Autodesk Fusion 360 part; units mm, degrees
sketch "Sketch1" plane through (0, 0, 0) normal (0, 1, 0) x (1, 0, 0)
  line L0 (39.5, -25.25) -> (-39.5, -25.25)
  line L1 (-43, -21.75) -> (-43, 21.75)
  line L2 (-39.5, 25.25) -> (39.5, 25.25)
  line L3 (43, 21.75) -> (43, -21.75)
  line L4 (-43, -25.25) -> (43, 25.25) construction
  arc A0 (-39.5, 25.25) -> (-43, 21.75) centre (-39.5, 21.75) ccw
  arc A1 (-43, -21.75) -> (-39.5, -25.25) centre (-39.5, -21.75) ccw
  arc A2 (43, 21.75) -> (39.5, 25.25) centre (39.5, 21.75) ccw
  arc A3 (39.5, -25.25) -> (43, -21.75) centre (39.5, -21.75) ccw
  line L5 (39, -21) -> (-39, -21) construction
  line L6 (-39, -21) -> (-39, 21) construction
  line L7 (-39, 21) -> (39, 21) construction
  line L8 (39, 21) -> (39, -21) construction
  line L9 (39, -21) -> (-39, 21) construction
  line L10 (-39, -21) -> (39, 21) construction
  circle A4 centre (39, -21) radius 1.6
  circle A5 centre (39, 21) radius 1.6
  circle A6 centre (-39, 21) radius 1.6
  circle A7 centre (-39, -21) radius 1.6
  dimension "d3" = 3.5
  dimension "d4" = 78
  dimension "d5" = 42
  dimension "d6" = 3.2
  dimension "d7" = 3.2
  dimension "d8" = 3.2
  dimension "d9" = 3.2
extrude "Extrude1" add sketch "Sketch1" along normal blind 1.6
sketch "Sketch2" plane through (0, 1.6, 0) normal (0, 1, 0) x (-1, 0, 0)
  circle A0 centre (-39, -21) radius 1.6
  circle A1 centre (39, 21) radius 1.6
  circle A2 centre (-39, 21) radius 1.6
  circle A3 centre (39, -21) radius 1.6
  arc A4 (43, 21.75) -> (39.5, 25.25) centre (39.5, 21.75) ccw
  line L0 (39.5, 25.25) -> (-39.5, 25.25)
  arc A5 (-39.5, 25.25) -> (-43, 21.75) centre (-39.5, 21.75) ccw
  line L1 (-43, 21.75) -> (-43, -21.75)
  arc A6 (-43, -21.75) -> (-39.5, -25.25) centre (-39.5, -21.75) ccw
  line L2 (-39.5, -25.25) -> (39.5, -25.25)
  arc A7 (39.5, -25.25) -> (43, -21.75) centre (39.5, -21.75) ccw
  line L3 (43, -21.75) -> (43, 21.75)
  line L4 (43, -25.25) -> (35, -25.25)
  line L5 (-43, -25.25) -> (-35, -25.25)
  line L6 (-35, -25.25) -> (-35, 25.25)
  line L7 (35, -25.25) -> (35, 25.25)
  dimension "d12" = 8
  dimension "d13" = 8
extrude "Extrude2" add sketch "Sketch2" along normal blind 4 contours L0 L2 L6 L7
sketch "Sketch3" plane through (0, 0, 0) normal (0, -1, 0) x (1, 0, 0)
  circle A0 centre (39, -21) radius 1.6
  circle A1 centre (-39, 21) radius 1.6
  circle A2 centre (39, 21) radius 1.6
  circle A3 centre (-39, -21) radius 1.6
  arc A4 (-39.5, 25.25) -> (-43, 21.75) centre (-39.5, 21.75) ccw
  line L0 (-43, 21.75) -> (-43, -21.75)
  arc A5 (-43, -21.75) -> (-39.5, -25.25) centre (-39.5, -21.75) ccw
  line L1 (-39.5, -25.25) -> (39.5, -25.25)
  arc A6 (39.5, -25.25) -> (43, -21.75) centre (39.5, -21.75) ccw
  line L2 (43, -21.75) -> (43, 21.75)
  arc A7 (43, 21.75) -> (39.5, 25.25) centre (39.5, 21.75) ccw
  line L3 (39.5, 25.25) -> (-39.5, 25.25)
  line L4 (43, 25.25) -> (13, 25.25)
  line L5 (13, 25.25) -> (-2, 25.25)
  line L6 (-2, 25.25) -> (-2, 10.25)
  line L7 (-2, 10.25) -> (13, 10.25)
  line L8 (13, 10.25) -> (13, 25.25)
  line L9 (13, 25.25) -> (-2, 25.25)
  line L10 (-2, 25.25) -> (-2, 28.25)
  line L11 (-2, 28.25) -> (13, 28.25)
  line L12 (13, 28.25) -> (13, 25.25)
  line L13 (43, 25.25) -> (43, 14.25)
  line L14 (43, 14.25) -> (37, 14.25)
  line L15 (37, 14.25) -> (37, 5.25)
  line L16 (37, 5.25) -> (43, 5.25)
  line L17 (43, 5.25) -> (43, 14.25)
  line L18 (43, 14.25) -> (44, 14.25)
  line L19 (44, 14.25) -> (44, 5.25)
  line L20 (44, 5.25) -> (43, 5.25)
  line L21 (43, 5.25) -> (43, 14.25)
  dimension "d16" = 30
  dimension "d17" = 15
  dimension "d18" = 15
  dimension "d19" = 3
  dimension "d20" = 11
  dimension "d21" = 6
  dimension "d22" = 9
  dimension "d23" = 1
  dimension "d24" = 9
extrude "Extrude3" add sketch "Sketch3" along normal blind 3 contours L3 L5 L9 L10 L11 L12 | L3 L5 L6 L7 L8 L9 | L2 L17 L18 L19 L20 L21 | L2 L14 L15 L16 L17 L21
Build history of the part. All positions in model axes, mm. A direction names the side the tool comes from. Round coordinates to 2 decimals unless told otherwise and drop trailing zeros. Loops run counter-clockwise (first coordinate to the right, second up) from the corner with the lowest first, then second, coordinate; pieces in that order, holes last.
Item 1: Which spindle directions (+Z, -Z, +X, -X, +Y, -Y) get a long thin tool onto all of the face, cutting with end or side? Do faces 4 (the face through (41, -1, 5.25)), 5 (the face through (35, 4, 0)), 6 (the face through (1, 3, 25.25)). Say none if no direction does.
Item 2: Saw through at B-B (z = 15.5). List the corners of the cut face in (x, y).
Item 3: Saw through at C-C (x = -20.5). List the corners of the cut face in (y, z).
Item 4: Saw through at A-A (y = -1.25). List the corners of the cut face in (x, z), then the cut area to 3 significant figures.
Item 5: Saw through at D-D (z = -2.5). List the corners of the cut face in (x, y).
Item 6: Drill centre lines: line 1 along Z through (x, y) = (39, 0.65); line 2 along X through (y, z) = (0.5, 21); line 3 along X through (y, z) = (3.25, -19). Where is each one in solid material? Low to high.
Item 7: Two-plate mould, pull along X, no slides. Class faces 1 (the face through (-39, 1.6, 0)), 2 (the face through (-39.208, 0.789, 22.586)), 3 (the face through (-43, 1, 0)): released by +X, released by -X, zero draft, split by the parting line, or undercut.
Item 8: Pin check, flat tips, straight feed: P1, Ø1.1, axis at x = 43.5, z = 8, coming from the +Y side; P2, Ø25, axis at x = -21, z = -8, coming from the -Y side; P3, Ø2, axis at y = 3.5, z = 7, coming from the +X side; P4, Ø3, axis at x = -39, z = -21, coming from the +Y side. Stop position of each tip, or through.
Worked answers:
1. face 4: -Z, +X, -X, -Y
1. face 5: +Z, -Z, +X, +Y
1. face 6: +Z, +X, -X, +Y
2. outline: (-43, 0) - (-2, 0) - (-2, -3) - (13, -3) - (13, 0) - (43, 0) - (43, 1.6) - (35, 1.6) - (35, 5.6) - (-35, 5.6) - (-35, 1.6) - (-43, 1.6) - close
3. outline: (0, -25.25) - (5.6, -25.25) - (5.6, 25.25) - (0, 25.25) - close
4. outline: (-2, 10.25) - (13, 10.25) - (13, 28.25) - (-2, 28.25) - close; (37, 5.25) - (44, 5.25) - (44, 14.25) - (37, 14.25) - close
4. area: 333 mm2
5. outline: (-43, 0) - (43, 0) - (43, 1.6) - (35, 1.6) - (35, 5.6) - (-35, 5.6) - (-35, 1.6) - (-43, 1.6) - close
6. line 1: z = -25.25 to -22.6, -19.4 to 19.4, 22.6 to 25.25
6. line 2: x = -43 to -40.6, -37.4 to 37.4, 40.6 to 43
6. line 3: x = -35 to 35
7. face 1: zero draft
7. face 2: undercut
7. face 3: released by -X
8. P1: stops at y = 1.6
8. P2: stops at y = 0
8. P3: stops at x = 35
8. P4: passes through
